Check sheet for the modelled part. Datum: model origin and axes. Units: mm. Face numbers are marked on the shaded views. A direction names the side the tool comes from. Give positions to 0.01 mm unless a question says otherwise; leave off trailing zeros. Order: outer loops, then holes, each group sorted by start corner. A loop starts at its lowest first (then second) coordinate and runs counter-clockwise, first axis right, second up. Notation, with made-up numbers: (-36.5, 89) -> (-3.5, 89) arc R35 cw to (-3.5, 128) -> close; hole circle Ø8 at (80.5, 88.25). An arc over 180 degrees is marked (long way). Answer in a Markdown table with one row per item. Add a question column.
(1) Cross-section at A-A (y = 2.5). Record the cut outline in (x, z), then the cut area to 3 significant figures.
(2) Cross-section at B-B (y = -12). Record the cut outline in (x, z).
(3) Thickness scan on L1, parallel to Y at x = 4.5, z = 0; L2, parallel to Z at x = 2.25, y = 17.5; L3, parallel to X at y = -13.5, z = -8.5. Record the ranges inside material, lowest first. Write a range as [from, to].
(4) Release check for a two-part mould opening along Y. For the marked faces 4, 5 and 6 record: released by +Y, released by -Y, zero draft, split by the parting line, or undercut.
(5) Go/stop test with flat-tipped pins: pin 1 (1.5 mm diameter, centred on x = 10.5, z = -10.5, fed in from +Y); pin 2 (1.5 mm diameter, centred on x = 5, z = 3, fed in from +Y); pin 3 (1 mm diameter, centred on x = 14, z = -12, fed in from +Y); pin 4 (2.5 mm diameter, centred on y = 0, z = 0, fed in from +X). Record where each tip stops, or that it passes through.
(6) Set-up check for the marked faces 1, 2 and 3: record each of +Z, -Z, +X, -X, +Y, -Y from which the full face is reachable in a straight line by a thin tool's end or side.
```python
from build123d import *

# Parameters (mm, degrees)
BASPROSKE_W     = 12
BASPROSKE_H     = 20.25
TOOTHCUT_DEPTH  = 32.050362317
TEETHCUTS_COUNT = 25
TEETHCUTS_ANGLE = 345.6
BORSKE_R        = 2
BORE_DEPTH      = 50.0000508
EXTRUDE_1_DEPTH = 5


with BuildPart() as part:
    # BasProSke → Base-Revolve (revolve)
    with BuildSketch(Plane(origin=(0, 0, 0), x_dir=(1, 0, 0), z_dir=(0, 1, 0)), mode=Mode.PRIVATE) as base_revolve_sk:
        with Locations((6, 10.125)):
            Rectangle(BASPROSKE_W, BASPROSKE_H)
    revolve(base_revolve_sk.sketch.rotate(Axis((-10, 0, 0), (1, 0, 0)), 180), axis=Axis((-10, 0, 0), (1, 0, 0)))

    # TooCutSke → ToothCut (cut, through all)
    with BuildSketch(Plane(origin=(0, 0, 0), x_dir=(0, 0, -1), z_dir=(1, 0, 0))):
        with BuildLine():
            ThreePointArc((0.713909619, 16.858891098), (0, 16.874), (-0.713909619, 16.858891098))
            ThreePointArc((-0.713909619, 16.858891098), (-1.221902209, 18.597177626), (-2.131751691, 20.163022588))
            ThreePointArc((-2.131751691, 20.163022588), (0, 20.2754), (2.131751691, 20.163022588))
            ThreePointArc((2.131751691, 20.163022588), (1.221902209, 18.597177626), (0.713909619, 16.858891098))
        make_face()
    toothcut = extrude(amount=TOOTHCUT_DEPTH, mode=Mode.SUBTRACT)

    # TeethCuts: ToothCut ×25 about axis
    teethcuts_axis = Axis((-10, 0, 0), (1, 0, 0))
    for i in range(1, TEETHCUTS_COUNT):
        add(toothcut.rotate(teethcuts_axis, i * TEETHCUTS_ANGLE / (TEETHCUTS_COUNT - 1)), mode=Mode.SUBTRACT)

    # BorSke → Bore (cut, symmetric)
    with BuildSketch(Plane(origin=(0, 0, 0), x_dir=(0, 0, -1), z_dir=(1, 0, 0))):
        with Locations(Location((0, 0, 0), (0, 0, 180))):
            Circle(BORSKE_R)
    extrude(amount=BORE_DEPTH, both=True, mode=Mode.SUBTRACT)

    # 草图2 → 凸台-拉伸1 (add)
    with BuildSketch(Plane(origin=(12, 0, 0), x_dir=(0, 0, -1), z_dir=(1, 0, 0))):
        with BuildLine():
            Line((-3.049889257, 6.851873869), (-5.083148762, 11.419789782))
            ThreePointArc((-5.083148762, 11.419789782), (0, 12.5), (5.083148762, 11.419789782))
            Line((5.083148762, 11.419789782), (3.049889257, 6.851873869))
            ThreePointArc((3.049889257, 6.851873869), (0, 7.5), (-3.049889257, 6.851873869))
        make_face()
        with BuildLine():
            Line((6.851873869, 3.049889257), (11.419789782, 5.083148762))
            ThreePointArc((11.419789782, 5.083148762), (12.5, 0), (11.419789782, -5.083148762))
            Line((11.419789782, -5.083148762), (6.851873869, -3.049889257))
            ThreePointArc((6.851873869, -3.049889257), (7.5, 0), (6.851873869, 3.049889257))
        make_face()
        with BuildLine():
            Line((3.049889257, -6.851873869), (5.083148762, -11.419789782))
            ThreePointArc((5.083148762, -11.419789782), (0, -12.5), (-5.083148762, -11.419789782))
            Line((-5.083148762, -11.419789782), (-3.049889257, -6.851873869))
            ThreePointArc((-3.049889257, -6.851873869), (0, -7.5), (3.049889257, -6.851873869))
        make_face()
        with BuildLine():
            Line((-6.851873869, -3.049889257), (-11.419789782, -5.083148762))
            ThreePointArc((-11.419789782, -5.083148762), (-12.5, 0), (-11.419789782, 5.083148762))
            Line((-11.419789782, 5.083148762), (-6.851873869, 3.049889257))
            ThreePointArc((-6.851873869, 3.049889257), (-7.5, 0), (-6.851873869, -3.049889257))
        make_face()
    extrude(amount=EXTRUDE_1_DEPTH)


solid = part.part
```
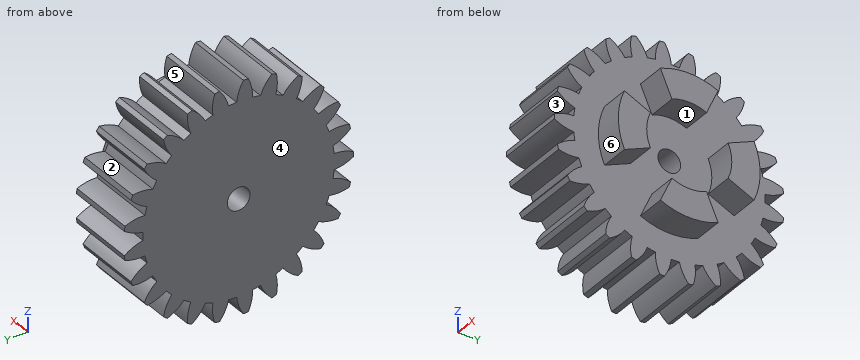
Answer below:
| question | item | result |
|---|---|---|
| 1 | outline | (0, -18.7) -> (12, -18.7) -> (12, -12.25) -> (17, -12.25) -> (17, -7.07) -> (12, -7.07) -> (12, 7.07) -> (17, 7.07) -> (17, 12.25) -> (12, 12.25) -> (12, 18.7) -> (0, 18.7) -> close |
| 1 | area | 501 mm² |
| 2 | outline | (0, -13.08) -> (12, -13.08) -> (12, -3.5) -> (17, -3.5) -> (17, 3.5) -> (12, 3.5) -> (12, 13.08) -> (0, 13.08) -> close |
| 3 | L1 | y = [-20.25, -2], [2, 16.87] |
| 3 | L2 | z = [-7.92, -5.65], [-3.52, -0.85], [0.85, 3.52], [5.65, 7.92] |
| 3 | L3 | x = [0, 12] |
| 4 | face 4 | zero draft |
| 4 | face 5 | undercut |
| 4 | face 6 | released by -Y |
| 5 | pin 1 | stops at y = 16.48 |
| 5 | pin 2 | stops at y = 20.12 |
| 5 | pin 3 | stops at y = 4.9 |
| 5 | pin 4 | passes through |
| 6 | face 1 | +X |
| 6 | face 2 | +X, -X |
| 6 | face 3 | +X, -X, -Y |
